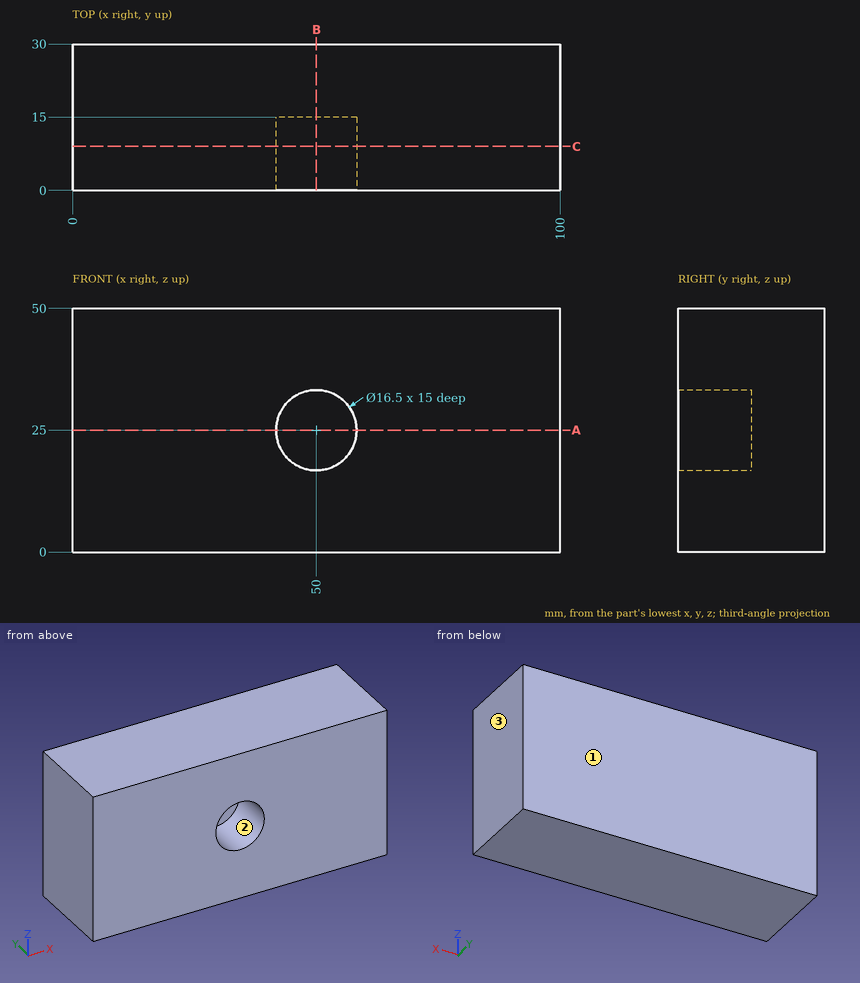
Can you work these out from the drawing? Everything is in mm from the part's minimum corner. Coordinates: 2 decimals unless noted, no trailing zeros. Loops run counter-clockwise (first coordinate to the right, second up) from the corner with the lowest first, then second, coordinate; pieces in that order, holes last.
1) Imagine slicing it at C-C (y = 9). List the corners of the cut face in (x, z) for me.
Reported:
outline: (0, 0) - (100, 0) - (100, 50) - (0, 50) - close; hole circle Ø16.5 at (50, 25)
2) Will this pin go through, and if not, where does the flat tip stop? pin 1 Ø5 at (x, z) = (47.5, 27.5) entering from -Y.
Reported:
pin 1: stops at y = 15
3) Please list where these lines run through material, in increasing order: line 1 along X through (y, z) = (12, 25); line 2 along Z through (x, y) = (50, 8.25); line 3 along Y through (x, z) = (51, 31).
Reported:
line 1: x = 0 to 41.75, 58.25 to 100
line 2: z = 0 to 16.75, 33.25 to 50
line 3: y = 15 to 30
4) Thinking about a two-plate mould opening in X: for the marked faces 1, 2 and 3, which applies, released by +X, released by -X, zero draft, split by the parting line, or undercut?
Reported:
face 1: zero draft
face 2: undercut
face 3: released by +X
5) Imagine slicing it at B-B (x = 50). List the corners of the cut face in (y, z) for me.
Reported:
outline: (0, 0) - (30, 0) - (30, 50) - (0, 50) - (0, 33.25) - (15, 33.25) - (15, 16.75) - (0, 16.75) - close
6) Imagine slicing it at A-A (z = 25). List the corners of the cut face in (x, y) for me.
Reported:
outline: (0, 0) - (41.75, 0) - (41.75, 15) - (58.25, 15) - (58.25, 0) - (100, 0) - (100, 30) - (0, 30) - close
